from build123d import *

# Parameters (mm, degrees)
FURO_ROSCADO_DE_M141_D           = 12
FURO_ROSCADO_DE_M141_DEPTH       = 50
FURO_ROSCADO_DE_M141_CSINK_D     = 14.05
FURO_ROSCADO_DE_M141_CSINK_ANGLE = 90
FURO_ROSCADO_DE_M141_TIP         = 3.605163714
FURO1_D                          = 9.68
FILETE1_R                        = 0.5
FILETE2_R                        = 1.5
CHANFRO1_SIZE                    = 0.5


with BuildPart() as part:
    # Esboço1 → Revolução1 (revolve)
    with BuildSketch(Plane.XY, mode=Mode.PRIVATE) as revolu_o1_sk:
        Polygon((0, 0), (63, 0), (63, 11), (53, 11), (53, 9.5), (48, 9.5), (48, 11), (5, 11), (5, 9.5), (0, 9.5), align=None)
    revolve(revolu_o1_sk.sketch.rotate(Axis((0, 0, 0), (1, 0, 0)), 90), axis=Axis((0, 0, 0), (1, 0, 0)))

    # Furo roscado de M141
    with Locations(Plane(origin=(63, 0, 0), x_dir=(0, 0, -1), z_dir=(1, 0, 0))):
        with Locations((0, 0)):
            CounterSinkHole(FURO_ROSCADO_DE_M141_D / 2, FURO_ROSCADO_DE_M141_CSINK_D / 2, depth=FURO_ROSCADO_DE_M141_DEPTH, counter_sink_angle=FURO_ROSCADO_DE_M141_CSINK_ANGLE)
            with Locations((0, 0, -(FURO_ROSCADO_DE_M141_DEPTH + FURO_ROSCADO_DE_M141_TIP / 2))):  # 118° drill point
                Cone(0, FURO_ROSCADO_DE_M141_D / 2, FURO_ROSCADO_DE_M141_TIP, mode=Mode.SUBTRACT)

    # Furo1 (through all)
    with Locations(Plane.ZY):
        with Locations((0, 0)):
            Hole(FURO1_D / 2)

    # Filete1
    filete1_edges = [part.edges().sort_by_distance(p)[0] for p in [
        (63, 0, -11),
        (0, 0, -9.5),
        (53, 0, -11),
    ]]
    fillet(filete1_edges, radius=FILETE1_R)

    # Filete2
    filete2_edges = [part.edges().sort_by_distance(p)[0] for p in [
        (0, 0, 4.84),
    ]]
    fillet(filete2_edges, radius=FILETE2_R)

    # Chanfro1
    chanfro1_edges = [part.edges().sort_by_distance(p)[0] for p in [
        (5, 0, -11),
        (48, 0, -11),
    ]]
    chamfer(chanfro1_edges, length=CHANFRO1_SIZE)


solid = part.part
Geometry check sheet. Reference: the model listing, model coordinates, mm. A direction names the side the tool comes from. Round coordinates to 2 decimals unless told otherwise and drop trailing zeros. Loops run counter-clockwise (first coordinate to the right, second up) from the corner with the lowest first, then second, coordinate; pieces in that order, holes last. Notation, with made-up numbers: (38.25, 32) - (89.25, 32) arc R16 ccw to (89.25, 38) - close; hole circle Ø9 at (37, -10.5). An arc over 180 degrees is marked (long way). One line per question, with ' | ' between items. Start each with the question number.
1. Depth check by flat-ended pin: pin 1 (6.5 mm diameter, centred on y = 3, z = -3.5, fed in from +X); pin 2 (12 mm diameter, centred on x = 6.5, z = -8.5, fed in from -Y); pin 3 (1 mm diameter, centred on x = 20.5, y = -2, fed in from +Z); pin 4 (10 mm diameter, centred on x = 42, z = 8, fed in from +Y). Enter the tip coordinate at first touch or a pass-through.
2. Scan lines: line 1 (X direction, y = 7.25, z = -6.5); line 2 (Y direction, x = 16.5, z = 0.25); line 3 (Y direction, x = 4, z = 0). Record each from-to range of solid material in increasing order. Write a range as [from, to].
3. Tool access check on faces 4 (the face through (63, 7, -2)), 5 (the face through (37, 0, -6)), 6 (the face through (2.718, 9.274, -2.059)), 7 (the face through (53, 9, -5)). Record the directions out of +Z, -Z, +X, -X, +Y, -Y that give a thin tool (end or side, any length) a straight path to the whole face; none if there is none.
4. Draft check along Y on faces 1 (the face through (7, 1.5, -4.6)), 2 (the face through (50.465, 9.274, -2.059)), 3 (the face through (48, 9, 5)). Enter one of: released by +Y, released by -Y, zero draft, split by the parting line, or undercut.
5. Cross-section at A-A on x = 40. Record the cut outline in (y, z).
Taken from the geometry:
1) pin 1: x = 63 | pin 2: y = -10.71 | pin 3: z = 10.9 | pin 4: y = 10.58
2) line 1: [5, 48], [53, 63] | line 2: [-11, -5.99], [5.99, 11] | line 3: [-9.5, -4.84], [4.84, 9.5]
3) face 4: +Z, -Z, +X, +Y, -Y | face 5: +X | face 6: -X | face 7: none
4) face 1: undercut | face 2: split by the parting line | face 3: zero draft
5) outline: circle Ø22 at (0, 0); hole circle Ø12 at (0, 0)
